Autodesk Inventor part; units mm, degrees
ref_plane "YZ Plane" through (0, 0, 0) normal (1, 0, 0) x (0, 1, 0)
ref_plane "XZ Plane" through (0, 0, 0) normal (0, 1, 0) x (-1, 0, 0)
ref_plane "XY Plane" through (0, 0, 0) normal (0, 0, 1) x (1, 0, 0)
sketch "スケッチ1" plane through (0, 0, 0) normal (1, 0, 0) x (0, 1, 0)
  line L0 (0, 0) -> (40, 69.282)
  line L1 (0, 0) -> (80, 0) construction
  line L2 (40, 69.282) -> (40, 0)
  line L3 (40, 0) -> (0, 0)
  dimension "d0" = 80
  dimension "d1" = 60
  dimension "d2" = 30
extrude "押し出し1" add sketch "スケッチ1" along normal blind 90
sketch "スケッチ2" plane through (0, 0, 0) normal (0, -0.866, 0.5) x (1, 0, 0)
  line L0 (0, 80) -> (10, 80)
  line L1 (10, 80) -> (10, 70)
  line L2 (10, 70) -> (0, 70)
  line L3 (0, 70) -> (0, 80)
  line L4 (90, 80) -> (80, 80)
  line L5 (80, 80) -> (80, 70)
  line L6 (80, 70) -> (90, 70)
  line L7 (90, 70) -> (90, 80)
  line L8 (90, 0) -> (80, 0)
  line L9 (80, 0) -> (80, 10)
  line L10 (80, 10) -> (90, 10)
  line L11 (90, 10) -> (90, 0)
  line L12 (0, 0) -> (10, 0)
  line L13 (10, 0) -> (10, 10)
  line L14 (10, 10) -> (0, 10)
  line L15 (0, 10) -> (0, 0)
  dimension "d5" = 10
  dimension "d6" = 10
  dimension "d7" = 10
  dimension "d8" = 10
  dimension "d9" = 10
  dimension "d10" = 10
  dimension "d11" = 10
  dimension "d12" = 10
hole "穴1" at (10, 35, 60.6218) at (10, 5, 8.6603) at (80, 5, 8.6603) at (80, 35, 60.6218) direction (0, 0.866, -0.5) diameter 2.5 depth 20 tip angle 118
sketch "スケッチ3" plane through (0, 0, 0) normal (0, 0, -1) x (-1, 0, 0)
  line L0 (-90, 40) -> (-75, 40)
  line L1 (-75, 40) -> (-75, 30)
  line L2 (-75, 30) -> (-90, 30)
  line L3 (-90, 30) -> (-90, 40)
  line L4 (-90, 0) -> (-75, 0)
  line L5 (-75, 0) -> (-75, 10)
  line L6 (-75, 10) -> (-90, 10)
  line L7 (-90, 10) -> (-90, 0)
  line L8 (0, 40) -> (-15, 40)
  line L9 (-15, 40) -> (-15, 30)
  line L10 (-15, 30) -> (0, 30)
  line L11 (0, 30) -> (0, 40)
  line L12 (0, 0) -> (-15, 0)
  line L13 (-15, 0) -> (-15, 10)
  line L14 (-15, 10) -> (0, 10)
  line L15 (0, 10) -> (0, 0)
  line L16 (-75, 30) -> (-15, 30)
  line L17 (-15, 10) -> (-75, 10)
  point P0 (-45, 10)
  point P1 (-45, 30)
  dimension "d20" = 15
  dimension "d21" = 10
  dimension "d23" = 15
  dimension "d24" = 10
  dimension "d25" = 15
  dimension "d26" = 10
hole "穴2" at (75, 30, 0) at (75, 10, 0) at (15, 30, 0) at (15, 10, 0) at (45, 10, 0) at (45, 30, 0) direction (0, 0, 1) diameter 2.5 depth 8 tip angle 118
sketch "スケッチ4" plane through (90, 0, 0) normal (1, 0, 0) x (0, 0, -1)
  line L0 (-69.282, 40) -> (0, 0)
  line L1 (0, 0) -> (0, 40)
  line L2 (0, 40) -> (-69.282, 40)
  line L3 (-8, 40) -> (-8, 4.6188)
  line L4 (0, 32) -> (-55.4256, 32)
  line L5 (-53.282, 40) -> (0, 9.2376)
  point P0 (-39.4256, 32)
  point P1 (-8, 32)
  point P2 (-8, 13.8564)
  dimension "d34" = 8
  dimension "d35" = 8
  dimension "d36" = 8
extrude "押し出し2" cut sketch "スケッチ4" against normal blind 35 contours L4 L3 L5
sketch "スケッチ5" plane through (0, 0, 0) normal (-1, 0, 0) x (0, 0, 1)
  line L0 (0, 0) -> (69.282, 40)
  line L1 (69.282, 40) -> (0, 40)
  line L2 (0, 40) -> (0, 0)
  line L3 (8, 40) -> (8, 33.1308)
  line L4 (8, 33.1308) -> (8, 4.6188)
  line L5 (0, 32) -> (55.2982, 32)
  line L6 (0, 9.2376) -> (53.282, 40)
  point P0 (39.4256, 32)
  point P1 (8, 32)
  point P2 (8, 13.8564)
  dimension "d39" = 8
  dimension "d40" = 8
  dimension "d41" = 8
extrude "押し出し3" cut sketch "スケッチ5" against normal blind 35 contours L4 L5 L6
properties part number "知能ロボコン土台"
For this review, take the finished solid that the model builds, in its own axes (mm). A direction names the side the tool comes from. Coordinates: 2 decimals unless noted, no trailing zeros. Write each loop counter-clockwise with the first axis right and the second up, starting at its lowest first coordinate (ties: lowest second). Pieces come first, ordered by that corner, then holes. Notation, with made-up numbers: (17, 22.5) - (30, 22.5) arc R26 cw to (30, 43.5) - close; hole circle Ø7 at (26.25, 29.25). An arc over 180 degrees is marked (long way). Answer in a Markdown table with one row per item. Add a question column.
Q1. Draft analysis for pull direction X (two halves, no side actions). For faces 4 (the cylindrical face through (14.155, 9.079, 4.056)), 5 (the flat face through (72.745, 23.055, 23.933)), 6 (the flat face through (35, 25, 20)), state which applies: +X half, -X half, draft (parallel to the pull), parting line (faces both ways), or undercut.
Q2. For P1, Ø1.5, axis at x = 75, y = 10, coming from the +Z side; P2, Ø3, axis at x = 15, y = 30, coming from the +Z side; P3, Ø4, axis at x = 13, z = 43, coming from the -Y side, all flat-tipped, find the tip position at first contact; note any pin that passes through.
Q3. We need section B-B, the plane x = 38.5. State the section outline as (y, z) points.
Q4. We need section A-A, the plane x = 64.5. State the section outline as (y, z) points, and give its area (3 significant figures).
Q5. For probe 1 along X at (y, z) = (10, 6); probe 2 along X at (y, z) = (10, 1.5); probe 3 along Y at (x, z) = (45, 3), list the stretches that pass through material, from the lowest coordinate up.
Q6. We need section C-C, the plane y = 27. State the section outline as (x, z) points, and give its area (3 significant figures).
Q7. Tool access review of faces 1 (the flat face through (55, 27, 17)), 2 (the flat face through (17, 32, 23)), 3 (the cylindrical face through (13.946, 30.672, 4.056)): name each direction out of +Z, -Z, +X, -X, +Y, -Y from which nothing blocks a thin tool from reaching the whole face with its end or side.
Q8. We need section D-D, the plane z = 44. State the section outline as (x, y) points, and give its area (3 significant figures).
Answer list:
| question | item | result |
|---|---|---|
| 1 | face 4 | undercut |
| 1 | face 5 | draft |
| 1 | face 6 | -X half |
| 2 | P1 | stops at z = 18.62 |
| 2 | P2 | stops at z = 54.56 |
| 2 | P3 | stops at y = 23.67 |
| 3 | outline | (0, 0) - (40, 0) - (40, 69.28) - close |
| 4 | outline | (0, 0) - (40, 0) - (40, 69.28) - close; hole (13.86, 8) - (32, 8) - (32, 39.43) - close |
| 4 | area | 1,100 mm2 |
| 5 | probe 1 | x = 0 to 8.77, 11.23 to 13.75, 16.25 to 43.75, 46.25 to 73.75, 76.25 to 78.77, 81.23 to 90 |
| 5 | probe 2 | x = 0 to 13.75, 16.25 to 43.75, 46.25 to 73.75, 76.25 to 90 |
| 5 | probe 3 | y = 1.73 to 8.75, 11.25 to 28.75, 31.25 to 40 |
| 6 | outline | (0, 0) - (90, 0) - (90, 8) - (55, 8) - (55, 30.77) - (90, 30.77) - (90, 46.77) - (0, 46.77) - (0, 30.77) - (35, 30.77) - (35, 8) - (0, 8) - close |
| 6 | area | 2,620 mm2 |
| 7 | face 1 | +X |
| 7 | face 2 | -X |
| 7 | face 3 | -Z |
| 8 | outline | (0, 25.4) - (90, 25.4) - (90, 40) - (0, 40) - close |
| 8 | area | 1,310 mm2 |
